Here's how the part is built. I have some questions about the finished solid (model axes, mm). Face numbers are marked on the shaded views. A direction names the side the tool comes from. Give positions to 0.01 mm unless a question says otherwise; leave off trailing zeros. Write each loop counter-clockwise with the first axis right and the second up, starting at its lowest first coordinate (ties: lowest second). Pieces come first, ordered by that corner, then holes. Notation, with made-up numbers: M 76.25,-15 L 100.25,-15 A27 cw 100.25,7 Z; hole C 79.5,39 d4. An arc over 180 degrees is marked long. Use one line per item in the form item = value. Start each with the question number.
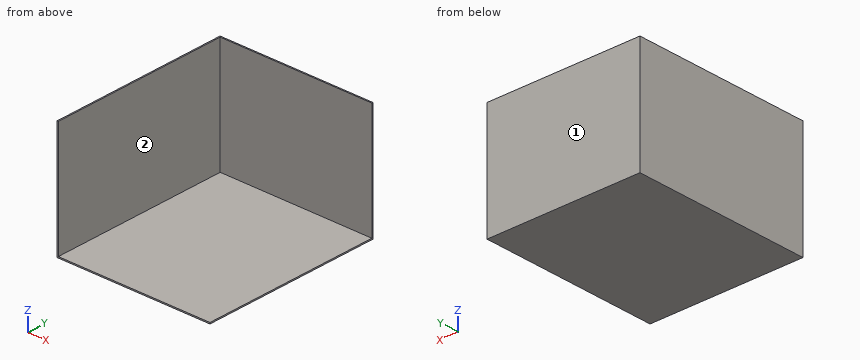
from build123d import *

# Parameters (mm, degrees)
F0_W     = 304.8
F0_H     = 355.6
F1_DEPTH = 228.6
F2_T     = -2.54


with BuildPart() as f1:
    # F0 (on Top) → F1 (new body)
    with BuildSketch(Plane.XY):
        with Locations((152.4, -177.8)):
            Rectangle(F0_W, F0_H)
    extrude(amount=F1_DEPTH)

    # F2
    f2_openings = [f1.faces().sort_by_distance(p)[0] for p in [
        (152.4, -177.8, 228.6),
        (152.4, -355.6, 114.3),
        (304.8, -177.8, 114.3),
    ]]
    offset(amount=F2_T, openings=f2_openings)


solid = f1.part
1) Will these pins go through, and if not, where does the flat tip stop? P1, Ø1, axis at x = 118.5, y = -236, coming from the +Z side; P2, Ø6, axis at y = -98, z = 124, coming from the +X side; P3, Ø1, axis at x = 103, z = 198, coming from the -Y side.
2) Please list where these lines run through material, in increasing order: line 1 (Y direction, x = 265, z = 119.5); line 2 (Z direction, x = 145, y = -49.5).
3) Suppose I cut it at A-A, the plane z = 200. List the corners of the cut face in (x, y) for me.
4) Suppose I cut it at B-B, the plane y = -128.5. List the corners of the cut face in (x, z) for me.
5) On a 3-axis mill with a long thin cutter (end or side, diameter ignored), from which of +Z, -Z, +X, -X, +Y, -Y can I reach the whole of each face in a straight line? I mean the marked faces 1 and 2. Say none if no direction works.
Checks:
q1.P1 = 2.54
q1.P2 = 2.54
q1.P3 = -2.54
q2.line_1 = -2.54 to 0
q2.line_2 = 0 to 2.54
q3.outline = M 0,-355.6 L 2.54,-355.6 L 2.54,-2.54 L 304.8,-2.54 L 304.8,0 L 0,0 Z
q4.outline = M 0,0 L 304.8,0 L 304.8,2.54 L 2.54,2.54 L 2.54,228.6 L 0,228.6 Z
q5.face_1 = +Z, -Z, +X, -X, +Y
q5.face_2 = +Z, +X, -Y
